from build123d import *

# Parameters (mm, degrees)
SKETCH_1_W          = 63.8
SKETCH_1_H          = 7.8
SKETCH_1_R          = 2.5
EXTRUDE_2_DEPTH     = 3.2
SKETCH_1_7_R        = 2.5
CUT_EXTRUDE_4_DEPTH = 1.8


with BuildPart() as part:
    # Sketch 1 → Extrude 2 (new body)
    # profile 1 of 9: a face of its own
    with BuildSketch(Plane(origin=(0, 0, 0), x_dir=(1, 0, 0), z_dir=(0, 1, 0))):
        Rectangle(SKETCH_1_W, SKETCH_1_H)
        with Locations((28, 0)):
            Circle(SKETCH_1_R, mode=Mode.SUBTRACT)
        with Locations((20, 0)):
            Circle(SKETCH_1_R, mode=Mode.SUBTRACT)
        with Locations((12, 0)):
            Circle(SKETCH_1_R, mode=Mode.SUBTRACT)
        with Locations((4, 0)):
            Circle(SKETCH_1_R, mode=Mode.SUBTRACT)
        with Locations((-4, 0)):
            Circle(SKETCH_1_R, mode=Mode.SUBTRACT)
        with Locations((-12, 0)):
            Circle(SKETCH_1_R, mode=Mode.SUBTRACT)
        with Locations((-20, 0)):
            Circle(SKETCH_1_R, mode=Mode.SUBTRACT)
        with Locations((-28, 0)):
            Circle(SKETCH_1_R, mode=Mode.SUBTRACT)
    # profile 2 of 9: a face of its own
    with BuildSketch(Plane(origin=(0, 0, 0), x_dir=(1, 0, 0), z_dir=(0, 1, 0))):
        with Locations((28, 0)):
            Circle(SKETCH_1_R)
    # profile 3 of 9: a face of its own
    with BuildSketch(Plane(origin=(0, 0, 0), x_dir=(1, 0, 0), z_dir=(0, 1, 0))):
        with Locations((20, 0)):
            Circle(SKETCH_1_R)
    # profile 4 of 9: a face of its own
    with BuildSketch(Plane(origin=(0, 0, 0), x_dir=(1, 0, 0), z_dir=(0, 1, 0))):
        with Locations((12, 0)):
            Circle(SKETCH_1_R)
    # profile 5 of 9: a face of its own
    with BuildSketch(Plane(origin=(0, 0, 0), x_dir=(1, 0, 0), z_dir=(0, 1, 0))):
        with Locations((4, 0)):
            Circle(SKETCH_1_R)
    # profile 6 of 9: a face of its own
    with BuildSketch(Plane(origin=(0, 0, 0), x_dir=(1, 0, 0), z_dir=(0, 1, 0))):
        with Locations((-4, 0)):
            Circle(SKETCH_1_R)
    # profile 7 of 9: a face of its own
    with BuildSketch(Plane(origin=(0, 0, 0), x_dir=(1, 0, 0), z_dir=(0, 1, 0))):
        with Locations((-12, 0)):
            Circle(SKETCH_1_R)
    # profile 8 of 9: a face of its own
    with BuildSketch(Plane(origin=(0, 0, 0), x_dir=(1, 0, 0), z_dir=(0, 1, 0))):
        with Locations((-20, 0)):
            Circle(SKETCH_1_R)
    # profile 9 of 9: a face of its own
    with BuildSketch(Plane(origin=(0, 0, 0), x_dir=(1, 0, 0), z_dir=(0, 1, 0))):
        with Locations((-28, 0)):
            Circle(SKETCH_1_R)
    extrude(amount=EXTRUDE_2_DEPTH)

    # Sketch 1_7 → Cut-Extrude 4 (cut)
    with BuildSketch(Plane(origin=(0, 0, 0), x_dir=(1, 0, 0), z_dir=(0, 1, 0))):
        with Locations(Location((-12, 0, 0), (0, 0, 270))):
            Circle(SKETCH_1_7_R)
        with Locations(Location((-4, 0, 0), (0, 0, 270))):
            Circle(SKETCH_1_7_R)
        with Locations(Location((12, 0, 0), (0, 0, 270))):
            Circle(SKETCH_1_7_R)
        with Locations(Location((20, 0, 0), (0, 0, 270))):
            Circle(SKETCH_1_7_R)
        with Locations(Location((28, 0, 0), (0, 0, 270))):
            Circle(SKETCH_1_7_R)
        with Locations(Location((-20, 0, 0), (0, 0, 270))):
            Circle(SKETCH_1_7_R)
        with Locations(Location((-28, 0, 0), (0, 0, 270))):
            Circle(SKETCH_1_7_R)
        with Locations(Location((4, 0, 0), (0, 0, 270))):
            Circle(SKETCH_1_7_R)
    extrude(amount=CUT_EXTRUDE_4_DEPTH, mode=Mode.SUBTRACT)


solid = part.part
Source: CAD feature listing. Evaluate the final solid. Frame: model axes, mm. A direction names the side the tool comes from. Round coordinates to 2 decimals unless told otherwise and drop trailing zeros. Loops run counter-clockwise (first coordinate to the right, second up) from the corner with the lowest first, then second, coordinate; pieces in that order, holes last. Notation, with made-up numbers: (66, 23) - (98, 23) arc R19 cw to (98, 54) - close; hole circle Ø8 at (-36, -14.5). An arc over 180 degrees is marked (long way). Write item = value, one per line. Start each with the question number.
(1) Pull-direction query (Z, two-part tool) for faces 1 (the face through (9.56, 0.89, -0.54)), 2 (the face through (0, 2, -3.9)), 3 (the face through (31.9, 2, 0)); classes: +Z half, -Z half, draft (parallel to the pull), parting line (faces both ways), or undercut.
(2) Ray query, line 1 along Z through (x, y) = (6, 0.85); line 2 along Y through (x, z) = (-11.5, -1); line 3 along Z through (x, y) = (-13, 1.1). Return the intervals inside material, ascending. Write a range as from..to.
(3) Section query A-A, the plane x = -28. Output: boundary loops of the cut face in (y, z), plus the area to 3 significant figures.
(4) Pin query (flat end, axial travel): pin 1 (1.5 mm diameter, centred on x = 4.5, z = 1, fed in from -Y). Return the tip coordinate at first contact, or that it passes through.
(5) Set-up query: faces 4 (the face through (-31.9, 2, 0)), 5 (the face through (-25.52, 0.89, -0.33)). Return all of +Z, -Z, +X, -X, +Y, -Y with unobstructed straight access to the full face (end or side cutting, diameter ignored); none if empty.
Conclusion:
q1.face_1 = undercut
q1.face_2 = -Z half
q1.face_3 = draft
q2.line_1 = -3.9..-1.5, 1.5..3.9
q2.line_2 = 1.8..3.2
q2.line_3 = -3.9..-2.29, 2.29..3.9
q3.outline = (0, -3.9) - (3.2, -3.9) - (3.2, 3.9) - (0, 3.9) - (0, 2.5) - (1.8, 2.5) - (1.8, -2.5) - (0, -2.5) - close
q3.area = 16.0 mm2
q4.pin_1 = 1.8
q5.face_4 = +Z, -Z, -X, +Y, -Y
q5.face_5 = -Y
